Here's how the part is built. I have some questions about the finished solid (model axes, mm). Coordinates: 2 decimals unless noted, no trailing zeros. Write each loop counter-clockwise with the first axis right and the second up, starting at its lowest first coordinate (ties: lowest second). Pieces come first, ordered by that corner, then holes.
```python
from build123d import *

# Parameters (mm, degrees)
SKETCH1_R           = 5
BOSS_EXTRUDE1_DEPTH = 6
SKETCH2_R           = 5
CUT_EXTRUDE1_DEPTH  = 436.529562716


with BuildPart() as part:
    # Sketch1 → Boss-Extrude1 (new body)
    with BuildSketch(Plane.XY):
        with BuildLine():
            Line((-425, -75), (-425, 35))
            ThreePointArc((-425, 35), (-419.142135624, 49.142135624), (-405, 55))
            Line((-405, 55), (-185.000330481, 55))
            ThreePointArc((-185.000330481, 55), (-177.92926267, 52.071067812), (-175.000330481, 45))
            Line((-175.000330481, 45), (-175.000330481, 25))
            ThreePointArc((-175.000330481, 25), (-172.071398293, 17.928932188), (-165.000330481, 15))
            Line((-165.000330481, 15), (-60, 15))
            ThreePointArc((-60, 15), (-52.928932188, 12.071067812), (-50, 5))
            Line((-50, 5), (-50, 0))
            ThreePointArc((-50, 0), (-35.355339059, -35.355339059), (0, -50))
            Line((0, -50), (0, -95))
            Line((0, -95), (-405, -95))
            ThreePointArc((-405, -95), (-419.142135624, -89.142135624), (-425, -75))
        make_face()
        with Locations((-350, 35)):
            Circle(SKETCH1_R, mode=Mode.SUBTRACT)
        with Locations((-275, 35)):
            Circle(SKETCH1_R, mode=Mode.SUBTRACT)
    boss_extrude1 = extrude(amount=BOSS_EXTRUDE1_DEPTH)

    # Mirror1: Boss-Extrude1 across plane
    add(boss_extrude1.mirror(Plane(origin=(0, -50, 6), x_dir=(0, 0, 1), z_dir=(-1, 0, 0))))

    # Sketch2 → Cut-Extrude1 (cut, through all)
    with BuildSketch(Plane.XY.offset(6)):
        with BuildLine():
            ThreePointArc((-310, -75), (-300, -65), (-290, -75))
            Line((-290, -75), (-290, -80))
            ThreePointArc((-290, -80), (-288.535533906, -83.535533906), (-285, -85))
            Line((-285, -85), (-115, -85))
            ThreePointArc((-115, -85), (-111.464466094, -83.535533906), (-110, -80))
            Line((-110, -80), (-110, -75))
            ThreePointArc((-110, -75), (-100, -65), (-90, -75))
            Line((-90, -75), (-90, -80))
            ThreePointArc((-90, -80), (-85, -85), (-80, -80))
            Line((-80, -80), (-80, 0))
            ThreePointArc((-80, 0), (-81.464466094, 3.535533906), (-85, 5))
            Line((-85, 5), (-165.000330481, 5))
            ThreePointArc((-165.000330481, 5), (-173.165296291, 6.742581416), (-179.907450331, 11.666666667))
            ThreePointArc((-179.907450331, 11.666666667), (-183.278527352, 14.128709292), (-187.361010256, 15))
            Line((-187.361010256, 15), (-405, 15))
            ThreePointArc((-405, 15), (-412.071067812, 12.071067812), (-415, 5))
            Line((-415, 5), (-415, -75))
            ThreePointArc((-415, -75), (-412.071067812, -82.071067812), (-405, -85))
            Line((-405, -85), (-315, -85))
            ThreePointArc((-315, -85), (-311.464466094, -83.535533906), (-310, -80))
            Line((-310, -80), (-310, -75))
        make_face()
        with BuildLine():
            ThreePointArc((-70, -80), (-68.535533906, -83.535533906), (-65, -85))
            Line((-65, -85), (0, -85))
            Line((0, -85), (0, -60))
            ThreePointArc((0, -60), (-42.426406871, -42.426406871), (-60, 0))
            Line((-60, 0), (-60, 5))
            Line((-60, 5), (-65, 5))
            ThreePointArc((-65, 5), (-68.535533906, 3.535533906), (-70, 0))
            Line((-70, 0), (-70, -80))
        make_face()
        with Locations((-300, -75)):
            Circle(SKETCH2_R)
        with Locations((-100, -75)):
            Circle(SKETCH2_R)
    cut_extrude1 = extrude(amount=-CUT_EXTRUDE1_DEPTH, mode=Mode.SUBTRACT)

    # Mirror2: Cut-Extrude1 across plane
    add(cut_extrude1.mirror(Plane(origin=(0, 0, 0), x_dir=(0, 0, 1), z_dir=(1, 0, 0))), mode=Mode.SUBTRACT)


solid = part.part
```
1) Imagine slicing it at B-B on y = -21.5. Please give me the cut outline in (x, z), then the cut area to 3 significant figures.
Values follow:
outline: (-425, 0) - (-415, 0) - (-415, 6) - (-425, 6) - close; (-80, 0) - (-70, 0) - (-70, 6) - (-80, 6) - close; (-56.02, 0) - (-45.14, 0) - (-45.14, 6) - (-56.02, 6) - close; (45.14, 0) - (56.02, 0) - (56.02, 6) - (45.14, 6) - close; (70, 0) - (80, 0) - (80, 6) - (70, 6) - close; (415, 0) - (425, 0) - (425, 6) - (415, 6) - close
area: 370 mm2
2) We'd pull the mould along X, two halves only. Please class faces 1 (the face through (-2, -53, 0)), 2 (the face through (-418.986, -89.297, 2.958)), 3 (the face through (419.297, 48.986, 2.958)): pulls with the +X half, pulls with the -X half, needs draft (parallel to the pull), parting line crosses it, or undercut.
Values follow:
face 1: needs draft
face 2: pulls with the -X half
face 3: pulls with the +X half
3) Imagine slicing it at A-A on x = -333. Please give me the cut outline in (y, z), then the cut area to 3 significant figures.
Values follow:
outline: (-95, 0) - (-85, 0) - (-85, 6) - (-95, 6) - close; (15, 0) - (55, 0) - (55, 6) - (15, 6) - close
area: 300 mm2
4) Imagine slicing it at C-C on z = 4.45. Count the separate pieces of the cut face and the enclosed holes in it, then the cut area to 3 significant figures.
Values follow:
separate pieces: 1
enclosed holes: 11
area: 37,300 mm2
5) I need wall thicknesses on probe 1 along Y at (x, z) = (300, 4.25); probe 2 along Y at (x, z) = (275, 1.45); probe 3 along Y at (x, z) = (-235, 2.1). Which ranges of each line are inside material? Lowest first, please.
Values follow:
probe 1: y = -95 to -80, -70 to -65, 15 to 55
probe 2: y = -95 to -85, 15 to 30, 40 to 55
probe 3: y = -95 to -85, 15 to 55
6) Will these pins go through, and if not, where does the flat tip stop? pin 1 (3 mm diameter, centred on x = 28.5, z = 4, fed in from +Y); pin 2 (13 mm diameter, centred on x = -100, y = -75, fed in from -Z); pin 3 (3 mm diameter, centred on x = -92, z = 4, fed in from +Y); pin 4 (1.5 mm diameter, centred on x = 25.5, z = 4, fed in from +Y).
Values follow:
pin 1: stops at y = -40
pin 2: stops at z = 0
pin 3: stops at y = 15
pin 4: stops at y = -42.56
